Autodesk Inventor part; units mm, degrees
ref_plane "YZ Plane" through (0, 0, 0) normal (1, 0, 0) x (0, 1, 0)
ref_plane "XZ Plane" through (0, 0, 0) normal (0, 1, 0) x (-1, 0, 0)
ref_plane "XY Plane" through (0, 0, 0) normal (0, 0, 1) x (1, 0, 0)
sketch "Skizze1" plane through (0, 0, 0) normal (1, 0, 0) x (0, 1, 0)
  line L0 (-30, -26) -> (30, -26)
  line L1 (30, -26) -> (24.2265, -16)
  line L2 (24.2265, -16) -> (32.5, -16)
  line L3 (32.5, -16) -> (32.5, 16)
  line L4 (32.5, 16) -> (-32.5, 16)
  line L5 (-32.5, 16) -> (-32.5, -16)
  line L6 (-32.5, -16) -> (-24.2265, -16)
  line L7 (-24.2265, -16) -> (-30, -26)
  point P0 (0, 0)
  dimension "d0" = 60
  dimension "d1" = 65
  dimension "d2" = 2.5
  dimension "d3" = 10
  dimension "d4" = 42
  dimension "d5" = 60
  dimension "d6" = 60
  dimension "d7" = 16
  dimension "d8" = 32.5
extrude "Extrusion1" add sketch "Skizze1" against normal blind 135
sketch "Skizze2" plane through (0, -32.5, 16) normal (0, 0, 1) x (1, 0, 0)
  line L0 (0, 0) -> (-135, 0)
  line L1 (-135, 0) -> (-85, 0)
  line L2 (-85, 0) -> (-85, 17.5)
  line L3 (-85, 17.5) -> (-135, 17.5)
  line L4 (-135, 17.5) -> (-135, 0)
  line L5 (-135, 65) -> (-135, 56.7265)
  line L6 (-135, 65) -> (-85, 65)
  line L7 (-85, 65) -> (-85, 47.5)
  line L8 (-85, 47.5) -> (-135, 47.5)
  line L9 (-135, 47.5) -> (-135, 65)
  point P0 (0, 32.5)
  point P1 (-85, 0)
  dimension "d11" = 50
  dimension "d12" = 17.5
  dimension "d13" = 50
  dimension "d14" = 17.5
extrude "Extrusion2" add sketch "Skizze2" along normal blind 43
fillet "Rundung1" radius 25 4 edges at (-85, -23.75, 59) (-135, -23.75, 59) (-85, 23.75, 59) (-135, 23.75, 59)
sketch "Skizze3" plane through (0, -32.5, -16) normal (0, -1, 0) x (1, 0, 0)
  line L0 (-85, 32) -> (-85, 50)
  line L1 (0, -10) -> (-135, -10)
  point P0 (0, 16)
  point P1 (-110, 50)
  dimension "d25" = 25
  dimension "d26" = 60
hole "Bohrung1" at (-110, -32.5, 34) direction (0, 1, 0) diameter 25 end through all
sketch "Skizze4" plane through (0, -32.5, 16) normal (0, 0, 1) x (1, 0, 0)
  line L0 (-55, 32.5) -> (-25, 32.5) construction
  line L1 (-55, 20) -> (-25, 20)
  line L2 (-25, 45) -> (-55, 45)
  arc A0 (-55, 45) -> (-55, 20) centre (-55, 32.5) ccw
  arc A1 (-25, 20) -> (-25, 45) centre (-25, 32.5) ccw
  line L3 (0, 65) -> (0, 0)
  line L4 (0, 0) -> (-85, 0)
  point P0 (0, 32.5)
  point P1 (-40, 32.5)
  dimension "d27" = 30
  dimension "d28" = 25
  dimension "d29" = 32.5
  dimension "d30" = 25
extrude "Extrusion3" cut sketch "Skizze4" against normal through all
sketch "Skizze5" plane through (0, -32.5, -16) normal (0, -1, 0) x (1, 0, 0)
  line L0 (-135, 77) -> (-85, 77)
  line L1 (-85, 77) -> (-85, 73)
  line L2 (-85, 73) -> (-135, 73)
  line L3 (-135, 73) -> (-135, 77)
  line L4 (-85, 32) -> (-85, 50)
  line L5 (-135, 0) -> (-135, 50)
  arc A0 (-85, 50) -> (-135, 50) centre (-110, 50) ccw
  point P0 (0, 16)
  point P1 (-110, 73)
  point P2 (-110, 75)
  dimension "d33" = 2
  dimension "d34" = 4
extrude "Extrusion4" cut sketch "Skizze5" against normal through all
sketch "Skizze6" plane through (-119.798, -32.5, 57) normal (0, 0, 1) x (1, 0, 0)
  line L0 (119.798, 65) -> (119.798, 0)
  line L1 (0, 65) -> (19.5959, 65)
  point P0 (119.798, 32.5)
  point P1 (9.798, 8.75)
  point P2 (9.798, 56.25)
  dimension "d44" = 110
  dimension "d45" = 110
  dimension "d46" = 47.5
  dimension "d47" = 8.75
hole "Bohrung2" at (-110, -23.75, 57) at (-110, 23.75, 57) direction (0, 0, -1) diameter 3.242 depth 14
chamfer "Fasen1" distance 0.5 angle 45 2 edges at (-110, 25.371, 57) (-110, -22.129, 57)
chamfer "Fasen2" distance 5 angle 45 2 edges at (0, -32.5, 0) (0, 32.5, 0)
properties part number "Schwalbenschwanzhalterung"
Work out the finished part from the listing and answer in its coordinate system (mm). A direction names the side the tool comes from. Round coordinates to 2 decimals unless told otherwise and drop trailing zeros. Write each loop counter-clockwise with the first axis right and the second up, starting at its lowest first coordinate (ties: lowest second). Pieces come first, ordered by that corner, then holes. Notation, with made-up numbers: M -16,26.5 L 13,26.5 A16 cw 13,37.5 Z; hole C 58.5,-12 d11. An arc over 180 degrees is marked long. Use a Markdown table: item, result.
1) Flat-ended cylindrical pins translate along their axes: pin 1 (4 mm diameter, centred on x = -110, y = 23.75, fed in from +Z); pin 2 (22.5 mm diameter, centred on x = -110, z = 34, fed in from +Y); pin 3 (1 mm diameter, centred on x = -68.5, y = 7.5, fed in from +Z); pin 4 (9 mm diameter, centred on y = -19.5, z = 27.5, fed in from +X). Find the tip coordinate at first contact, or state that the pin passes through.
Taken from the geometry:
| item | result |
|---|---|
| pin 1 | stops at z = 56.88 |
| pin 2 | passes through |
| pin 3 | stops at z = 16 |
| pin 4 | stops at x = -85 |
2) Determine the mould class of faces 1 (the face through (-89.26, -23.63, 47.96)), 2 (the face through (-113.755, -23.627, 22.077)), 3 (the face through (-2.5, 30, -0.2)) for opening direction Z: pulls with the +Z half, pulls with the -Z half, needs draft (parallel to the pull), parting line crosses it, or undercut.
Taken from the geometry:
| item | result |
|---|---|
| face 1 | pulls with the +Z half |
| face 2 | undercut |
| face 3 | needs draft |
3) Consider line 1 (Y direction, x = -110, z = 53); line 2 (Y direction, x = -43, z = -6); line 3 (X direction, y = -26.25, z = 34). Determine where each line is inside the solid, lowest interval first. Write a range as [from, to].
Taken from the geometry:
| item | result |
|---|---|
| line 1 | y = [-32.5, -25.37], [-22.13, -15], [15, 22.13], [25.37, 32.5] |
| line 2 | y = [-32.5, -12.5], [12.5, 32.5] |
| line 3 | x = [-135, -122.5], [-97.5, -85] |
4) The part is cut by section B-B on z = -7. Give the vertices of the cut face in (x, y).
Taken from the geometry:
| item | result |
|---|---|
| outline | M -135,-32.5 L -5,-32.5 L 0,-27.5 L 0,27.5 L -5,32.5 L -135,32.5 Z; hole M -55,-12.5 L -25,-12.5 A12.5 ccw -25,12.5 L -55,12.5 A12.5 ccw Z |
5) The part is cut by section A-A on x = -110. State how many separate pieces and enclosed holes the cut face has, plus the area to 3 significant figures.
Taken from the geometry:
| item | result |
|---|---|
| separate pieces | 5 |
| enclosed holes | 0 |
| area | 3,110 mm2 |
6) The part is cut by section C-C on y = 0. Give the vertices of the cut face in (x, z), plus the area to 3 significant figures.
Taken from the geometry:
| item | result |
|---|---|
| outline | M -135,-26 L -67.5,-26 L -67.5,16 L -135,16 Z; M -12.5,-26 L 0,-26 L 0,16 L -12.5,16 Z |
| area | 3,360 mm2 |
7) Which of the six approach directions +Z, -Z, +X, -X, +Y, -Y give full straight-line access (tool end or side, diameter ignored) to faces 4 (the face through (-85, -24, 25)), 5 (the face through (-66.555, -27.073, -20.93)), 6 (the face through (-104.1, 15, 45.3))?
Taken from the geometry:
| item | result |
|---|---|
| face 4 | +Z, +X, +Y, -Y |
| face 5 | +X, -X, -Y |
| face 6 | +Z, +X, -X |
8) The part is cut by section D-D on x = -32. Give the vertices of the cut face in (y, z), plus the area to 3 significant figures.
Taken from the geometry:
| item | result |
|---|---|
| outline | M -32.5,-16 L -24.23,-16 L -30,-26 L -12.5,-26 L -12.5,16 L -32.5,16 Z; M 12.5,-26 L 30,-26 L 24.23,-16 L 32.5,-16 L 32.5,16 L 12.5,16 Z |
| area | 1,570 mm2 |
